Here's the drawing with two shaded views (mm, measured from the low corner). I have some questions. Coordinates: 2 decimals unless noted, no trailing zeros. Loops run counter-clockwise (first coordinate to the right, second up) from the corner with the lowest first, then second, coordinate; pieces in that order, holes last.
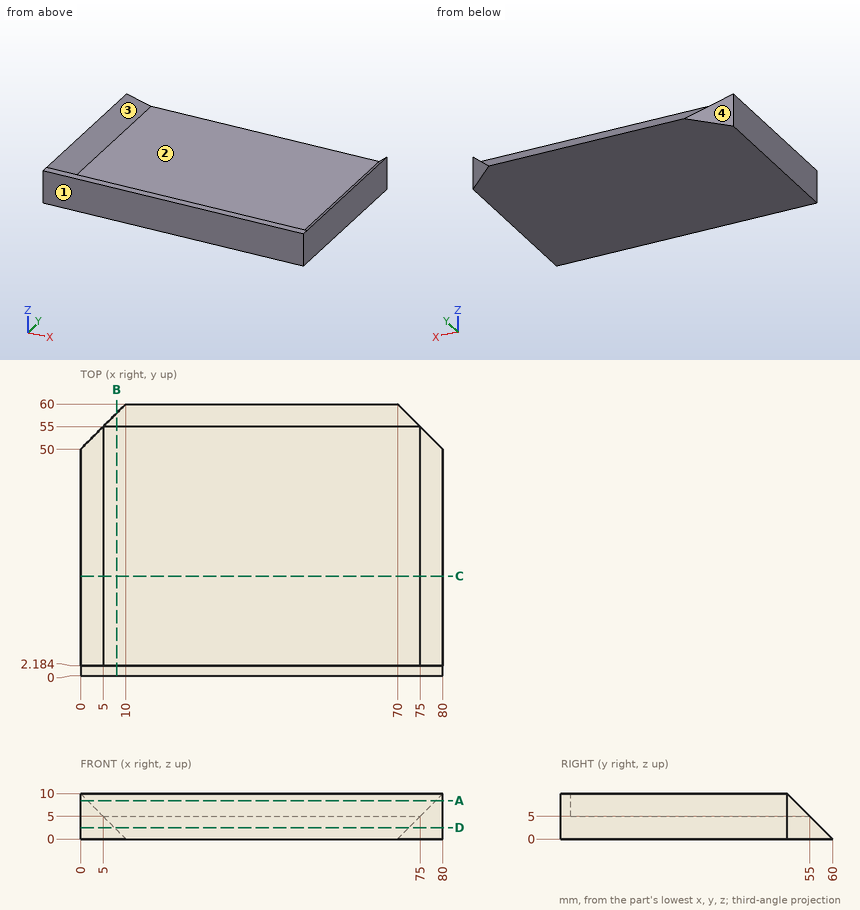
(1) I want a section at D-D on z = 2.5. Write out the boundary of the cut face in (x, y), then the cut area to 3 significant figures.
Check values:
outline: (0, 0) - (80, 0) - (80, 50) - (72.5, 57.5) - (7.5, 57.5) - (0, 50) - close
area: 4,540 mm2
(2) I want a section at B-B on x = 8. Write out the boundary of the cut face in (y, z).
Check values:
outline: (0, 0) - (58, 0) - (58, 2) - (55, 5) - (2.18, 5) - (2.18, 10) - (0, 10) - close
(3) I want a section at C-C on y = 22. Write out the boundary of the cut face in (x, z), then the cut area to 3 significant figures.
Check values:
outline: (0, 0) - (80, 0) - (80, 10) - (75, 5) - (5, 5) - (0, 10) - close
area: 425 mm2
(4) I want a section at A-A on z = 8.5. Write out the boundary of the cut face in (x, y).
Check values:
outline: (0, 0) - (80, 0) - (80, 50) - (78.5, 51.5) - (78.5, 2.18) - (1.5, 2.18) - (1.5, 51.5) - (0, 50) - close
(5) If we mould it in two halves opening along X, with no side actions, what happens to the marked faces 1, 2, 3 and 4? For each: released by +X, released by -X, zero draft, split by the parting line, or undercut.
Check values:
face 1: zero draft
face 2: undercut
face 3: undercut
face 4: released by -X
(6) I'm going to push flat-ended pins straight in: pin 1 (2 mm diameter, centred on x = 37.5, z = 3.5, fed in from +Y); pin 2 (4 mm diameter, centred on x = 41.5, z = 8.5, fed in from +Y); pin 3 (4 mm diameter, centred on x = 67, y = 23, fed in from +Z). Where does each tip first touch, or does it pass through?
Check values:
pin 1: stops at y = 57.5
pin 2: stops at y = 2.18
pin 3: stops at z = 5
(7) If I drill on probe 1 along Z at (x, y) = (27, 9.5); probe 2 along Y at (x, z) = (48, 7.5); probe 3 along X at (y, z) = (16, 6.25), over which ranges is the centre line in solid material (lowest first)?
Check values:
probe 1: z = 0 to 5
probe 2: y = 0 to 2.18
probe 3: x = 0 to 3.75, 76.25 to 80
